```python
from build123d import *

# Parameters (mm, degrees)
ESQUISSE1_R                  = 13.715
ESQUISSE1_R_2                = 4
BASE_EXTRUSION_DEPTH         = 10
ENL_V_MAT_EXTRU_1_DEPTH      = 28.860410083
R_P_TITION_CIRCULAIRE1_COUNT = 18
ENL_V_START                  = -1.25
ESQUISSE3_R                  = 13.715
ESQUISSE3_R_2                = 10
ENL_V_MAT_EXTRU_2_DEPTH      = 1.25
ESQUISSE4_R                  = 13.715
ESQUISSE4_R_2                = 10
ENL_V_MAT_EXTRU_3_DEPTH      = 1.25


with BuildPart() as part:
    # Esquisse1 → Base-Extrusion (new, symmetric)
    with BuildSketch(Plane.XY):
        Circle(ESQUISSE1_R)
        Circle(ESQUISSE1_R_2, mode=Mode.SUBTRACT)
    extrude(amount=BASE_EXTRUSION_DEPTH, both=True)

    # Esquisse2 → Enlèv. mat.-Extru.1 (cut, through all)
    with BuildSketch(Plane.XY.offset(10)):
        with BuildLine():
            Line((0.878200621, 11.96782201), (1.646660653, 13.615789867))
            ThreePointArc((1.646660653, 13.615789867), (-0.120274569, 13.714472612), (-1.885207275, 13.584815734))
            Line((-1.885207275, 13.584815734), (-1.121695723, 11.947459927))
            ThreePointArc((-1.121695723, 11.947459927), (-0.1221725, 11.999378062), (0.878200621, 11.96782201))
        make_face()
    enl_v_mat_extru_1 = extrude(amount=-ENL_V_MAT_EXTRU_1_DEPTH, mode=Mode.SUBTRACT)

    # Répétition circulaire1: Enlèv. mat.-Extru.1 ×18 about axis
    r_p_tition_circulaire1_axis = Axis((0, 0, 0), (0, 0, 1))
    for i in range(1, R_P_TITION_CIRCULAIRE1_COUNT):
        add(enl_v_mat_extru_1.rotate(r_p_tition_circulaire1_axis, i * 360 / R_P_TITION_CIRCULAIRE1_COUNT), mode=Mode.SUBTRACT)

    # Esquisse3 → Enlèv. mat.-Extru.2 (cut)
    with BuildSketch(Plane(origin=(0, 0, -10), x_dir=(-1, 0, 0), z_dir=(0, 0, -1)).offset(ENL_V_START)):
        Circle(ESQUISSE3_R)
        Circle(ESQUISSE3_R_2, mode=Mode.SUBTRACT)
    extrude(amount=ENL_V_MAT_EXTRU_2_DEPTH, mode=Mode.SUBTRACT)

    # Esquisse4 → Enlèv. mat.-Extru.3 (cut)
    with BuildSketch(Plane.XY.offset(10)):
        Circle(ESQUISSE4_R)
        with Locations(Location((0, 0, 0), (0, 0, 180))):
            Circle(ESQUISSE4_R_2, mode=Mode.SUBTRACT)
    extrude(amount=-ENL_V_MAT_EXTRU_3_DEPTH, mode=Mode.SUBTRACT)


solid = part.part
```
Input: part model. Units: mm. Frame: model coordinates. A direction names the side the tool comes from. Coordinates: 2 decimals unless noted, no trailing zeros. Order: outer loops, then holes, each group sorted by start corner. A loop starts at its lowest first (then second) coordinate and runs counter-clockwise, first axis right, second up. Notation, with made-up numbers: (4.5, 21) - (10.5, 21) arc R17 ccw to (10.5, 53) - close; hole circle Ø10 at (42, 87.5). An arc over 180 degrees is marked (long way). Put each result on its own line as item: value.
1. Cut plane B-B on x = 0. Return the cut outline in (y, z), then the cut area to 3 significant figures.
Report:
outline: (-12, -8.75) - (-10, -8.75) - (-10, -10) - (-4, -10) - (-4, 10) - (-10, 10) - (-10, 8.75) - (-12, 8.75) - close; (4, -10) - (10, -10) - (10, -8.75) - (12, -8.75) - (12, 8.75) - (10, 8.75) - (10, 10) - (4, 10) - close
area: 310 mm2
2. Contact query for flat-ended pins moving along their axis: pin 1 Ø5 at (x, z) = (-2.5, 7.5) entering from +Y; pin 2 Ø6.5 at (x, y) = (0, 0) entering from +Z; pin 3 Ø4 at (x, z) = (8.5, -5) entering from -Y; pin 4 Ø3 at (y, z) = (9, 6.5) entering from -X. Output: stop coordinate, or through.
Report:
pin 1: stops at y = 13.58
pin 2: passes through
pin 3: stops at y = -12.08
pin 4: stops at x = -10.97
3. Reachability of faces 1 (the face through (-9.37, 8.82, 0.12)), 2 (the face through (10.44, -7.48, 0.12)), 3 (the face through (5.788, -11.491, 0.123)) from +Z, -Z, +X, -X, +Y, -Y: full face, straight path, thin tool, end or side. Return the list, or none.
Report:
face 1: +Z, -Z, +Y
face 2: +Z, -Z, +X
face 3: +Z, -Z, -Y
4. Cut plane C-C on y = 6.25. Return the cut outline in (x, z), then the cut area to 3 significant figures.
Report:
outline: (-10.24, -8.75) - (-7.81, -8.75) - (-7.81, -10) - (7.81, -10) - (7.81, -8.75) - (10.24, -8.75) - (10.24, 8.75) - (7.81, 8.75) - (7.81, 10) - (-7.81, 10) - (-7.81, 8.75) - (-10.24, 8.75) - close
area: 398 mm2
5. Draft query along Y for faces 4 (the face through (-11.793, -2.218, 0.123)), 5 (the face through (2.272, 13.526, 0.123)), 6 (the face through (4.23, -11.23, 0.12)). Return one class per face: pulls with the +Y half, pulls with the -Y half, needs draft (parallel to the pull), parting line crosses it, or undercut.
Report:
face 4: undercut
face 5: pulls with the +Y half
face 6: pulls with the -Y half
6. Line query: line 1 along Y through (x, z) = (0, 2.25); line 2 along Z through (x, y) = (6.25, -11.25); line 3 along Y through (x, z) = (0.75, 5.25). Output: solid intervals per line, ascending.
Report:
line 1: y = -12 to -4, 4 to 12
line 2: z = -8.75 to 8.75
line 3: y = -11.98 to -3.93, 3.93 to 11.98
7. Cut plane A-A on y = 0. Return the cut outline in (x, z) (3 decimals), then the cut area to 3 significant figures.
Report:
outline: (-13.715, -8.75) - (-10, -8.75) - (-10, -10) - (-4, -10) - (-4, 10) - (-10, 10) - (-10, 8.75) - (-13.715, 8.75) - close; (4, -10) - (10, -10) - (10, -8.75) - (13.715, -8.75) - (13.715, 8.75) - (10, 8.75) - (10, 10) - (4, 10) - close
area: 370 mm2
